Build history of the part. All positions in model axes, mm. A direction names the side the tool comes from. Give positions to 0.01 mm unless a question says otherwise; leave off trailing zeros. Loops run counter-clockwise (first coordinate to the right, second up) from the corner with the lowest first, then second, coordinate; pieces in that order, holes last. Notation, with made-up numbers: M 27.5,31 L 45.5,31 A23 cw 45.5,68 Z; hole C 26,25.25 d10. An arc over 180 degrees is marked long. Put each result on its own line as item: value.
```python
from build123d import *

# Parameters (mm, degrees)
SKETCH2_R                      = 9.5
SKETCH2_R_2                    = 8.3
CUT_EXTRUDE1_REACH             = 267.847
CUT_EXTRUDE1_DIRECTION_2_REACH = 267.847
CUT_EXTRUDE2_REACH             = 267.847
CUT_EXTRUDE2_END_RADIUS        = 9.5
SKETCH4_R                      = 4


with BuildPart() as part:
    # Sweep1: sweep along a path in Sketch1
    with BuildLine(Plane.XY) as sweep1_path:
        Line((-21.6, 0), (0, 0))
        Line((0, 0), (185.373442264, 0))
        ThreePointArc((185.373442264, 0), (218.798397967, -12.165688958), (236.58344542, -42.970294761))
        Line((236.58344542, -42.970294761), (240.75, -66.6))
        Line((240.75, -66.6), (243.236210428, -80.7))
    # Sketch2 → Sweep1 (sweep)
    with BuildSketch(Plane.ZY.offset(21.6)):
        Circle(SKETCH2_R)
        Circle(SKETCH2_R_2, mode=Mode.SUBTRACT)
    sweep(path=sweep1_path.line)

    # Sketch3 → Cut-Extrude1 (cut, up to next)
    with BuildSketch(Plane.XY, mode=Mode.PRIVATE) as cut_extrude1_sk1:
        with BuildLine():
            Line((245.149518391, -67.939949686), (244.425905183, -63.836135257))
            ThreePointArc((244.425905183, -63.836135257), (243.809058208, -62.867879457), (242.688221287, -62.619395894))
            Line((242.688221287, -62.619395894), (237.567220972, -63.522366418))
            ThreePointArc((237.567220972, -63.522366418), (236.598965172, -64.139213393), (236.350481609, -65.260050314))
            Line((236.350481609, -65.260050314), (237.074094817, -69.363864743))
            ThreePointArc((237.074094817, -69.363864743), (237.690941792, -70.332120543), (238.811778713, -70.580604106))
            Line((238.811778713, -70.580604106), (243.932779028, -69.677633582))
            ThreePointArc((243.932779028, -69.677633582), (244.901034828, -69.060786607), (245.149518391, -67.939949686))
        make_face()
    cut_extrude1_tool1 = extrude(cut_extrude1_sk1.sketch, amount=-CUT_EXTRUDE1_REACH, mode=Mode.PRIVATE) & part.part
    add(cut_extrude1_tool1.solids().sort_by_distance((240.75, -66.6, 0))[0], mode=Mode.SUBTRACT)

    # Sketch3 → Cut-Extrude1 direction 2 (cut, up to next)
    with BuildSketch(Plane.XY, mode=Mode.PRIVATE) as cut_extrude1_direction_2_sk1:
        with BuildLine():
            Line((245.149518391, -67.939949686), (244.425905183, -63.836135257))
            ThreePointArc((244.425905183, -63.836135257), (243.809058208, -62.867879457), (242.688221287, -62.619395894))
            Line((242.688221287, -62.619395894), (237.567220972, -63.522366418))
            ThreePointArc((237.567220972, -63.522366418), (236.598965172, -64.139213393), (236.350481609, -65.260050314))
            Line((236.350481609, -65.260050314), (237.074094817, -69.363864743))
            ThreePointArc((237.074094817, -69.363864743), (237.690941792, -70.332120543), (238.811778713, -70.580604106))
            Line((238.811778713, -70.580604106), (243.932779028, -69.677633582))
            ThreePointArc((243.932779028, -69.677633582), (244.901034828, -69.060786607), (245.149518391, -67.939949686))
        make_face()
    cut_extrude1_direction_2_tool1 = extrude(cut_extrude1_direction_2_sk1.sketch, amount=CUT_EXTRUDE1_DIRECTION_2_REACH, mode=Mode.PRIVATE) & part.part
    add(cut_extrude1_direction_2_tool1.solids().sort_by_distance((240.75, -66.6, 0))[0], mode=Mode.SUBTRACT)

    # Cut-Extrude2: up to this cylinder (the profile starts inside it)
    cut_extrude2_end = Plane(origin=(0, 0, 0), z_dir=(-1, 0, 0)) * Cylinder(CUT_EXTRUDE2_END_RADIUS, 555.694, mode=Mode.PRIVATE)
    # Sketch4 → Cut-Extrude2 (cut, up to the surface)
    with BuildSketch(Plane.XY, mode=Mode.PRIVATE) as cut_extrude2_sk1:
        with Locations(Location((0, 0, 0), (0, 0, 90))):
            Circle(SKETCH4_R)
    cut_extrude2_tool1 = extrude(cut_extrude2_sk1.sketch, amount=CUT_EXTRUDE2_REACH, mode=Mode.PRIVATE) & cut_extrude2_end
    add(cut_extrude2_tool1.solids().sort_by_distance((0, 0, 0))[0], mode=Mode.SUBTRACT)


solid = part.part
```
Q1. Tool access for faces 1 (the cylindrical face through (-3.966, -0.521, 8.618)), 2 (the flat face through (-21.6, 6, -6)): list every direction of +Z, -Z, +X, -X, +Y, -Y with a clear straight run to the whole face (end or side of a thin tool).
Here are the results:
face 1: +Z
face 2: +Z, -Z, -X, +Y, -Y
Q2. Drop flat-ended pins along their axis: pin 1 Ø10 at (x, z) = (91.5, 3.5) entering from +Y; pin 2 Ø6 at (y, z) = (-33, 0.5) entering from +X; pin 3 Ø4 at (y, z) = (-20, -3.5) entering from -X; pin 4 Ø5 at (x, z) = (157.5, 2.5) entering from -Y. Give the stop position or say it passes through.
Here are the results:
pin 1: y = 9.5
pin 2: x = 244.75
pin 3: x = 211.73
pin 4: y = -9.5
Q3. Slice it at B-B (x = 80). List the corners of the cut face in (y, z), and give its area (3 significant figures).
Here are the results:
outline: C 0,0 d19; hole C 0,0 d16.6
area: 67.1 mm²
Q4. Slice it at A-A (z = 0.25). List the corners of the cut face in (x, y), and give its area (3 significant figures).
Here are the results:
outline: M -21.6,-9.5 L 185.37,-9.5 A42.5 cw 227.23,-44.62 L 233.88,-82.35 L 235.07,-82.14 L 228.41,-44.41 A43.7 ccw 185.37,-8.3 L -21.6,-8.3 Z; M -21.6,8.3 L 185.37,8.3 A60.3 cw 244.75,-41.53 L 251.41,-79.26 L 252.59,-79.05 L 245.94,-41.32 A61.5 ccw 185.37,9.5 L -21.6,9.5 Z
area: 763 mm²
Q5. Probe line 1 (Y direction, x = 121.5, z = 0); line 2 (Y direction, x = 187.5, z = 3.25). List the from-to ranges inside material, lowest first. Write a range as from..to.
Here are the results:
line 1: -9.5..-8.3, 8.3..9.5
line 2: -8.98..-7.69, 7.6..8.89
Q6. Slice it at C-C (x = 0). List the corners of the cut face in (y, z).
Here are the results:
outline: M -4,7.27 L -4,8.62 A9.5 ccw long 4,8.62 L 4,7.27 A8.3 cw long Z
Q7. Mould opens along Z. For faces 3 (the cylindrical face through (83.336, 3.639, 8.776)), 4 (the cylindrical face through (83.336, 8.103, -1.799)), 5 (the flat face through (248.044, -79.852, 6.993)) say: pulls with the +Z half, pulls with the -Z half, needs draft (parallel to the pull), parting line crosses it, or undercut.
Here are the results:
face 3: parting line crosses it
face 4: undercut
face 5: needs draft
